Geometry: final body of the model. Coordinates: model frame, mm. Face numbers are marked on the shaded views. A direction names the side the tool comes from. Give positions to 0.01 mm unless a question says otherwise; leave off trailing zeros. Order: outer loops, then holes, each group sorted by start corner. A loop starts at its lowest first (then second) coordinate and runs counter-clockwise, first axis right, second up. Notation, with made-up numbers: M 48.25,7 L 80.25,7 A17 cw 80.25,25 Z; hole C 42,-23.75 d11. An arc over 180 degrees is marked long. Write item = value, one per line. Start each with the question number.
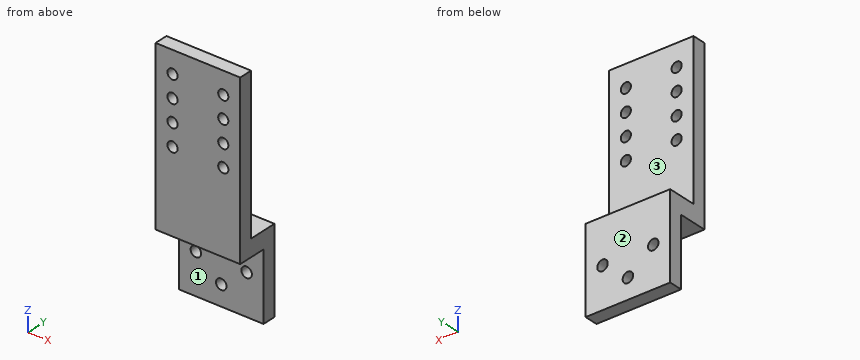
from build123d import *

# Parameters (mm, degrees)
SKETCH_1_W          = 25
SKETCH_1_H          = 70
SKETCH_1_R          = 1.55
SKETCH_1_R_2        = 1.5
EXTRUDE_1_DEPTH     = 4
SKETCH_2_W          = 25
SKETCH_2_H          = 25
SKETCH_2_R          = 1.55
EXTRUDE_2_DEPTH     = 8.6
SKETCH_3_W          = 25
SKETCH_3_H          = 20
SKETCH_3_R          = 1.55
CUT_EXTRUDE_1_DEPTH = 8.6


with BuildPart() as part:
    # Эскиз1 → Бобышка-Вытянуть1 (new body)
    with BuildSketch(Plane(origin=(0, 0, 0), x_dir=(1, 0, 0), z_dir=(0, 1, 0))):
        with Locations((0, 13.852233677)):
            Rectangle(SKETCH_1_W, SKETCH_1_H)
        with Locations((-7.5, 36.852233677)):
            Circle(SKETCH_1_R, mode=Mode.SUBTRACT)
        with Locations((7.5, 36.852233677)):
            Circle(SKETCH_1_R, mode=Mode.SUBTRACT)
        with Locations((-7.5, -14.647766323)):
            Circle(SKETCH_1_R_2, mode=Mode.SUBTRACT)
        with Locations((7.5, -14.647766323)):
            Circle(SKETCH_1_R_2, mode=Mode.SUBTRACT)
        with Locations((-7.5, -8.147766323)):
            Circle(SKETCH_1_R_2, mode=Mode.SUBTRACT)
        with Locations((7.5, -8.147766323)):
            Circle(SKETCH_1_R_2, mode=Mode.SUBTRACT)
        with Locations((-7.5, -1.647766323)):
            Circle(SKETCH_1_R_2, mode=Mode.SUBTRACT)
        with Locations((7.5, -1.647766323)):
            Circle(SKETCH_1_R_2, mode=Mode.SUBTRACT)
        with Locations((-7.5, 4.852233677)):
            Circle(SKETCH_1_R_2, mode=Mode.SUBTRACT)
        with Locations((7.5, 4.852233677)):
            Circle(SKETCH_1_R_2, mode=Mode.SUBTRACT)
        with Locations((0, 42.852233677)):
            Circle(SKETCH_1_R, mode=Mode.SUBTRACT)
    extrude(amount=EXTRUDE_1_DEPTH)

    # Эскиз2 → Бобышка-Вытянуть2 (add)
    with BuildSketch(Plane(origin=(0, 4, 0), x_dir=(1, 0, 0), z_dir=(0, 1, 0))):
        with Locations((0, 36.352233677)):
            Rectangle(SKETCH_2_W, SKETCH_2_H)
        with Locations((0, 42.852233677)):
            Circle(SKETCH_2_R, mode=Mode.SUBTRACT)
        with Locations((7.5, 36.852233677)):
            Circle(SKETCH_2_R, mode=Mode.SUBTRACT)
        with Locations((-7.5, 36.852233677)):
            Circle(SKETCH_2_R, mode=Mode.SUBTRACT)
    extrude(amount=EXTRUDE_2_DEPTH)

    # Эскиз3 → Вырез-Вытянуть1 (cut)
    with BuildSketch(Plane.XZ):
        with Locations((0, -38.852233677)):
            Rectangle(SKETCH_3_W, SKETCH_3_H)
        with Locations((-7.5, -36.852233677)):
            Circle(SKETCH_3_R, mode=Mode.SUBTRACT)
        with Locations((7.5, -36.852233677)):
            Circle(SKETCH_3_R, mode=Mode.SUBTRACT)
        with Locations((0, -42.852233677)):
            Circle(SKETCH_3_R, mode=Mode.SUBTRACT)
    extrude(amount=-CUT_EXTRUDE_1_DEPTH, mode=Mode.SUBTRACT)


solid = part.part
1) Cut plane C-C (z = 2.5). Return loops of the section in (x, y), plus the area to 4 significant figures.
2) Cut plane D-D (z = -12). Return loops of the section in (x, y), plus the area to 3 significant figures.
3) Cut plane A-A (x = -7.5). Return loops of the section in (y, z), plus the area to 3 significant figures.
4) Ray query, L1, parallel to Z at x = -7.5, y = 2.55; L2, parallel to Y at x = 1, z = 5; L3, parallel to Z at x = 3, y = 4.75. Return the intervals inside material, ascending.
5) Pin query (flat end, axial travel): pin 1 Ø2.5 at (x, z) = (-7.5, 14.65) entering from +Y; pin 2 Ø6 at (x, y) = (5, 7.5) entering from +Z; pin 3 Ø12 at (x, z) = (0, 9) entering from +Y; pin 4 Ø4 at (x, y) = (-4.5, 2.5) entering from -Z. Return the tip coordinate at first contact, or that it passes through.
6) Access query for the marked faces 1, 2 and 3. Directions: +Z, -Z, +X, -X, +Y, -Y. A direction counts if a zero-diameter tool reaches every point of the face in a straight line with its end or side. Return the directions, or none.
7) Cut plane B-B (x = 0). Return loops of the section in (y, z).
Reply:
q1.outline = M -12.5,0 L -8.73,0 L -8.73,4 L -12.5,4 Z; M -6.27,0 L 6.27,0 L 6.27,4 L -6.27,4 Z; M 8.73,0 L 12.5,0 L 12.5,4 L 8.73,4 Z
q1.area = 80.25 mm²
q2.outline = M -12.5,0 L 12.5,0 L 12.5,4 L -12.5,4 Z
q2.area = 100 mm²
q3.outline = M 0,-28.85 L 8.6,-28.85 L 8.6,-35.3 L 12.6,-35.3 L 12.6,-23.85 L 4,-23.85 L 4,-6.35 L 0,-6.35 Z; M 0,-3.35 L 4,-3.35 L 4,0.15 L 0,0.15 Z; M 0,3.15 L 4,3.15 L 4,6.65 L 0,6.65 Z; M 0,9.65 L 4,9.65 L 4,13.15 L 0,13.15 Z; M 0,16.15 L 4,16.15 L 4,21.15 L 0,21.15 Z; M 8.6,-48.85 L 12.6,-48.85 L 12.6,-38.4 L 8.6,-38.4 Z
q3.area = 263 mm²
q4.L1 = -28.85 to -6.35, -3.35 to 0.15, 3.15 to 6.65, 9.65 to 13.15, 16.15 to 21.15
q4.L2 = 0 to 4
q4.L3 = -28.85 to -23.85
q5.pin_1 = through
q5.pin_2 = -23.85
q5.pin_3 = 4
q5.pin_4 = -28.85
q6.face_1 = -Z, +X, -X, -Y
q6.face_2 = +Z, -Z, +X, -X, +Y
q6.face_3 = +Z, +X, -X, +Y
q7.outline = M 0,-28.85 L 8.6,-28.85 L 8.6,-41.3 L 12.6,-41.3 L 12.6,-23.85 L 4,-23.85 L 4,21.15 L 0,21.15 Z; M 8.6,-48.85 L 12.6,-48.85 L 12.6,-44.4 L 8.6,-44.4 Z
